Build history of the part. All positions in model axes, mm. Face numbers are marked on the shaded views. A direction names the side the tool comes from. Round coordinates to 2 decimals unless told otherwise and drop trailing zeros. Loops run counter-clockwise (first coordinate to the right, second up) from the corner with the lowest first, then second, coordinate; pieces in that order, holes last. Notation, with made-up numbers: M 43,53 L 64,53 A25 cw 64,86 Z; hole C -40,40 d1. An arc over 180 degrees is marked long. One line per item, written item: value.
```python
from build123d import *

# Parameters (mm, degrees)
SKETCH001_R  = 17.29
PAD_DEPTH    = 3
CHAMFER_SIZE = 0.5


with BuildPart() as part:
    # Sketch → Revolution (revolve)
    with BuildSketch(Plane.XZ):
        Polygon((-19.4, 0), (-19.4, 2.831371), (-17.29, 4.941371), (-17.29, 10), (-16.49, 10), (-16.49, 4.61), (-18.6, 2.5), (-18.6, 0), align=None)
    revolve(axis=Axis((0, 0, 0), (0, 0, 1)))

    # Sketch001 (on DatumPlane) → Pad (new body)
    with BuildSketch(Plane.XY.offset(10)):
        Circle(SKETCH001_R)
        with BuildLine():
            ThreePointArc((-6.631907, 11.631907), (-10.16744, 10.16744), (-11.631907, 6.631907))
            Line((-11.631907, -6.631907), (-11.631907, 6.631907))
            ThreePointArc((-11.631907, -6.631907), (-10.16744, -10.16744), (-6.631907, -11.631907))
            Line((6.631907, -11.631907), (-6.631907, -11.631907))
            ThreePointArc((6.631907, -11.631907), (10.16744, -10.16744), (11.631907, -6.631907))
            Line((11.631907, 6.631907), (11.631907, -6.631907))
            ThreePointArc((11.631907, 6.631907), (10.16744, 10.16744), (6.631907, 11.631907))
            Line((-6.631907, 11.631907), (6.631907, 11.631907))
        make_face(mode=Mode.SUBTRACT)
    extrude(amount=PAD_DEPTH)

    # Chamfer
    chamfer_edges = [part.edges().sort_by_distance(p)[0] for p in [
        (0, -11.631907, 10),
        (10.16744, -10.16744, 10),
        (-10.16744, -10.16744, 10),
        (-11.631907, 0, 10),
        (11.631907, 0, 10),
        (10.16744, 10.16744, 10),
        (0, 11.631907, 10),
        (-10.16744, 10.16744, 10),
        (0, -11.631907, 13),
        (10.16744, -10.16744, 13),
        (11.631907, 0, 13),
        (10.16744, 10.16744, 13),
        (0, 11.631907, 13),
        (-10.16744, 10.16744, 13),
        (-11.631907, 0, 13),
        (-10.16744, -10.16744, 13),
        (0, 17.29, 13),
        (0, -17.29, 13),
    ]]
    chamfer(chamfer_edges, length=CHAMFER_SIZE)


solid = part.part
```
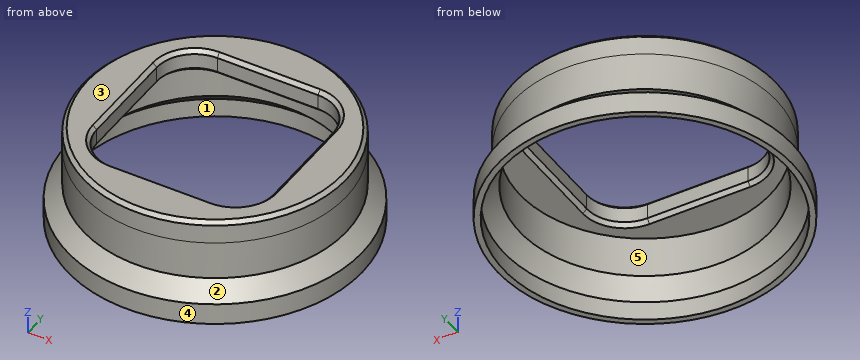
Item 1: Slice it at D-D, the plane z = 8. Give the cut face in (x, y), and give its area (3 significant figures).
Check values:
outline: C 0,0 d34.58; hole C 0,0 d32.98
area: 84.9 mm2
Item 2: Pull direction X, two halves, no side cores. Call the marked faces 3, 4 and 5: pulls with the +X half, pulls with the -X half, needs draft (parallel to the pull), parting line crosses it, or undercut.
Check values:
face 3: needs draft
face 4: parting line crosses it
face 5: undercut
Item 3: Slice it at B-B, the plane z = 11.5. Give the cut face in (x, y).
Check values:
outline: C 0,0 d34.58; hole M -11.63,-6.63 A5 ccw -6.63,-11.63 L 6.63,-11.63 A5 ccw 11.63,-6.63 L 11.63,6.63 A5 ccw 6.63,11.63 L -6.63,11.63 A5 ccw -11.63,6.63 Z
Item 4: Slice it at A-A, the plane x = 0. Give the cut face in (y, z), and give its area (3 significant figures).
Check values:
outline: M -19.4,0 L -18.6,0 L -18.6,2.5 L -16.49,4.61 L -16.49,10 L -12.13,10 L -11.63,10.5 L -11.63,12.5 L -12.13,13 L -16.79,13 L -17.29,12.5 L -17.29,4.94 L -19.4,2.83 Z; M 11.63,10.5 L 12.13,10 L 16.49,10 L 16.49,4.61 L 18.6,2.5 L 18.6,0 L 19.4,0 L 19.4,2.83 L 17.29,4.94 L 17.29,12.5 L 16.79,13 L 12.13,13 L 11.63,12.5 Z
area: 50.6 mm2
Item 5: Wall check: line 1 along X through (y, z) = (0, 7.9); line 2 along Y through (x, z) = (0, 1.05). Give the ranges that are in metal, low to high.
Check values:
line 1: x = -17.29 to -16.49, 16.49 to 17.29
line 2: y = -19.4 to -18.6, 18.6 to 19.4
Item 6: Drop flat-ended pins along their axis: P1, Ø1, axis at x = -2.5, z = 2.5, coming from the -Y side; P2, Ø1.5, axis at y = 2, z = 1.5, coming from the -X side; P3, Ø0.6, axis at y = -3.5, z = 11.5, coming from the +X side; P4, Ø4, axis at x = -12, y = -5, coming from the +Z side. Give the stop position or say it passes through.
Check values:
P1: stops at y = -19.3
P2: stops at x = -19.36
P3: stops at x = 16.99
P4: stops at z = 13
Item 7: Which spindle directions (+Z, -Z, +X, -X, +Y, -Y) get a long thin tool onto all of the face, cutting with end or side? Do the marked faces 1 and 2. Say none if no direction does.
Check values:
face 1: -Z
face 2: +Z
